Model file for the job. Use its own axes, mm. A direction names the side the tool comes from. Coordinates: 2 decimals unless noted, no trailing zeros. Order: outer loops, then holes, each group sorted by start corner. A loop starts at its lowest first (then second) coordinate and runs counter-clockwise, first axis right, second up. Notation, with made-up numbers: (-24.5, 0.25) -> (4.5, 0.25) arc R34 cw to (4.5, 36.25) -> close; hole circle Ø10 at (73.5, 39.25). An arc over 180 degrees is marked (long way). Use CSV: the item, a comma, the result in double quotes. Start each with the question number.
(1) Cut at A-A on x = 0. Write the cut outline in (y, z), plus the area to 3 significant figures.
(2) Pin check, flat tips, straight feed: pin 1 Ø5 at (x, z) = (-4, -14) entering from +Y; pin 2 Ø3 at (x, z) = (0, 4) entering from +Y; pin 3 Ø3 at (x, y) = (-3.5, 0.5) entering from -Z; pin 4 Ø1 at (x, y) = (-3, 2) entering from +Z. Stop position of each tip, or through.
(3) Tool access for faces 1 (the cylindrical face through (-1.517, 3.021, 6.834)), 2 (the cylindrical face through (0.05, 2.46, -5.25)): list every direction of +Z, -Z, +X, -X, +Y, -Y with a clear straight run to the whole face (end or side of a thin tool).
(4) Cut at C-C on z = 4. Write the cut outline in (x, y), plus the area to 3 significant figures.
(5) Pull direction X, two halves, no side cores. Call faces 3 (the cylindrical face through (-5.22, 2.46, -0.27)), 4 (the cylindrical face through (0, 2, -27)), 5 (the flat face through (0, 0, -10)): pulls with the +X half, pulls with the -X half, needs draft (parallel to the pull), parting line crosses it, or undercut.
(6) Cut at B-B on y = 1.4. Write the cut outline in (x, z).
(7) Cut at D-D on x = 4.75. Write the cut outline in (y, z), plus the area to 3 significant figures.
(8) Probe L1, parallel to X at y = 2.6, z = 0; L2, parallel to X at y = 1.15, z = -4; L3, parallel to Y at x = -0.25, z = -15. List the from-to ranges inside material, lowest first.
```python
from build123d import *

# Parameters (mm, degrees)
SKETCH_1_R      = 1.25
SKETCH_1_R_2    = 3
EXTRUDE_1_DEPTH = 4
CHAMFER_1_SIZE  = 1
SKETCH_2_R      = 7
SKETCH_2_R_2    = 1.25
EXTRUDE_2_DEPTH = 1


with BuildPart() as part:
    # 草图1 → 凸台-拉伸1 (new body)
    with BuildSketch(Plane(origin=(0, 0, 0), x_dir=(1, 0, 0), z_dir=(0, 1, 0))):
        with BuildLine():
            Line((-7, 0), (-7, 20))
            ThreePointArc((-7, 20), (0, 27), (7, 20))
            Line((7, 20), (7, 0))
            ThreePointArc((7, 0), (0, -7), (-7, 0))
        make_face()
        with Locations(Location((0, 4, 0), (0, 0, 270))):
            Circle(SKETCH_1_R, mode=Mode.SUBTRACT)
        with Locations(Location((4, 0, 0), (0, 0, 270))):
            Circle(SKETCH_1_R, mode=Mode.SUBTRACT)
        with Locations(Location((0, -4, 0), (0, 0, 270))):
            Circle(SKETCH_1_R, mode=Mode.SUBTRACT)
        with Locations(Location((-4, 0, 0), (0, 0, 270))):
            Circle(SKETCH_1_R, mode=Mode.SUBTRACT)
        with Locations(Location((0, 20, 0), (0, 0, 270))):
            Circle(SKETCH_1_R_2, mode=Mode.SUBTRACT)
    extrude(amount=EXTRUDE_1_DEPTH)

    # 倒角1
    chamfer_1_edges = [part.edges().sort_by_distance(p)[0] for p in [
        (0, 4, -23),
    ]]
    chamfer(chamfer_1_edges, length=CHAMFER_1_SIZE)

    # 草图2 → 凸台-拉伸2 (add)
    with BuildSketch(Plane(origin=(0, 4, 0), x_dir=(1, 0, 0), z_dir=(0, 1, 0))):
        Circle(SKETCH_2_R)
        with Locations(Location((4, 0, 0), (0, 0, 270))):
            Circle(SKETCH_2_R_2, mode=Mode.SUBTRACT)
        with Locations(Location((0, 4, 0), (0, 0, 270))):
            Circle(SKETCH_2_R_2, mode=Mode.SUBTRACT)
        with Locations(Location((-4, 0, 0), (0, 0, 270))):
            Circle(SKETCH_2_R_2, mode=Mode.SUBTRACT)
        with Locations(Location((0, -4, 0), (0, 0, 270))):
            Circle(SKETCH_2_R_2, mode=Mode.SUBTRACT)
    extrude(amount=EXTRUDE_2_DEPTH)


solid = part.part
```
Outcome:
1,outline,"(0, -27) -> (4, -27) -> (4, -24) -> (3, -23) -> (0, -23) -> close; (0, -17) -> (3, -17) -> (4, -16) -> (4, -7) -> (5, -7) -> (5, -5.25) -> (0, -5.25) -> close; (0, -2.75) -> (5, -2.75) -> (5, 2.75) -> (0, 2.75) -> close; (0, 5.25) -> (5, 5.25) -> (5, 7) -> (0, 7) -> close"
1,area,"100 mm2"
2,pin 1,"y = 4"
2,pin 2,"y = 5"
2,pin 3,"z = -26.71"
2,pin 4,"z = 6.54"
3,face 1,"+Y"
3,face 2,"+Y, -Y"
4,outline,"(-5.74, 0) -> (-1.25, 0) -> (-1.25, 5) -> (-5.74, 5) -> close; (1.25, 0) -> (5.74, 0) -> (5.74, 5) -> (1.25, 5) -> close"
4,area,"44.9 mm2"
5,face 3,"undercut"
5,face 4,"parting line crosses it"
5,face 5,"needs draft"
6,outline,"(-7, -20) arc R7 ccw to (7, -20) -> (7, 0) arc R7 ccw to (-7, 0) -> close; hole circle Ø2.5 at (-4, 0); hole circle Ø6 at (0, -20); hole circle Ø2.5 at (0, -4); hole circle Ø2.5 at (0, 4); hole circle Ø2.5 at (4, 0)"
7,outline,"(0, -25.14) -> (4, -25.14) -> (4, -5.14) -> (5, -5.14) -> (5, -1) -> (0, -1) -> close; (0, 1) -> (5, 1) -> (5, 5.14) -> (0, 5.14) -> close"
7,area,"121 mm2"
8,L1,"-7 to -5.25, -2.75 to 2.75, 5.25 to 7"
8,L2,"-7 to -1.25, 1.25 to 7"
8,L3,"0 to 4"
